Source: CAD feature listing. Evaluate the final solid. Frame: model axes, mm. Face numbers are marked on the shaded views. Round coordinates to 2 decimals unless told otherwise and drop trailing zeros. Loops run counter-clockwise (first coordinate to the right, second up) from the corner with the lowest first, then second, coordinate; pieces in that order, holes last. Notation, with made-up numbers: (66.5, -16.75) - (125.5, -16.75) arc R19 cw to (125.5, 8.25) - close; hole circle Ø10 at (29, -27). An arc over 180 degrees is marked (long way). Write item = value, one per line. Start each with the question number.
from build123d import *

# Parameters (mm, degrees)
F0_W      = 80
F0_H      = 120
F0_R      = 2.5
F0_R_2    = 1
F1_DEPTH  = 50
F3_DEPTH  = 120.001
F5_R      = 5
F6_DEPTH  = 10
F7_R      = 7.5
F8_DEPTH  = 120
F13_R     = 1
F15_DEPTH = 94.020238
F14_R     = 1
F16_DEPTH = 94.020238


with BuildPart() as f1:
    # F0 (on Front) → F1 (new body)
    with BuildSketch(Plane.XZ):
        Rectangle(F0_W, F0_H)
        with Locations((0, -50)):
            Circle(F0_R, mode=Mode.SUBTRACT)
        with Locations((0, 30)):
            Circle(F0_R, mode=Mode.SUBTRACT)
        with Locations((0, 45)):
            Circle(F0_R_2, mode=Mode.SUBTRACT)
    extrude(amount=F1_DEPTH)

    # F2 (on face) → F3 (cut, through all)
    with BuildSketch(Plane(origin=(0, 0, -60), x_dir=(1, 0, 0), z_dir=(0, 0, -1))):
        with BuildLine():
            Line((43.30127, 50), (-43.30127, 50))
            ThreePointArc((-43.30127, 50), (0, 25), (43.30127, 50))
        make_face()
    extrude(amount=-F3_DEPTH, mode=Mode.SUBTRACT)

    # F5 (on offset) → F6 (cut)
    with BuildSketch(Plane.XZ.offset(30)):
        with Locations((0, -50)):
            Circle(F5_R)
        with Locations((0, 30)):
            Circle(F5_R)
    extrude(amount=-F6_DEPTH, mode=Mode.SUBTRACT)

    # F7 (on face) → F8 (cut, through all)
    with BuildSketch(Plane(origin=(0, 0, -60), x_dir=(1, 0, 0), z_dir=(0, 0, -1))):
        with Locations((-17.5, 12)):
            Circle(F7_R)
        with Locations((17.5, 12)):
            Circle(F7_R)
    extrude(amount=-F8_DEPTH, mode=Mode.SUBTRACT)

    # F13 (on face) → F15 (cut, through all)
    with BuildSketch(Plane(origin=(17.524047, 30.35254, 0), x_dir=(-0.866025, 0.5, 0), z_dir=(0.5, 0.866025, 0))):
        with Locations((-37.5, 45)):
            Circle(F13_R)
    extrude(amount=-F15_DEPTH, mode=Mode.SUBTRACT)

    # F14 (on face) → F16 (cut, through all)
    with BuildSketch(Plane(origin=(-17.524047, 30.35254, 0), x_dir=(-0.866025, -0.5, 0), z_dir=(-0.5, 0.866025, 0))):
        with Locations((37.5, 45)):
            Circle(F14_R)
    extrude(amount=-F16_DEPTH, mode=Mode.SUBTRACT)


solid = f1.part
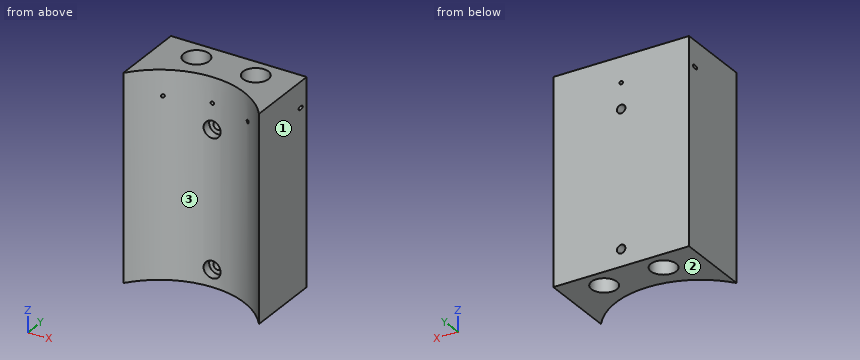
(1) Cut plane D-D (y = -17). State how many separate pieces and enclosed holes the cut face has, and give its area (3 significant figures).
(2) Material intervals for line 1 along Z through (x, y) = (0, -23); line 2 along X through (y, z) = (-11, 30); line 3 along X through (y, z) = (-21.15, -50), sorted ascending. Write a range as from..to.
(3) Cut plane B-B (z = -9.5). Output: boundary loops of the cut face in (x, y).
(4) Cut plane C-C (x = -15). Output: boundary loops of the cut face in (y, z), and give its area (3 significant figures).
(5) Mould query, pull axis X, two halves, no side actions, for the marked faces 1, 2 and 3. Classes: +X half, -X half, draft (parallel to the pull), parting line (faces both ways), or undercut.
(6) Pin query (flat end, axial travel): P1, Ø12, axis at x = -29, z = -19, coming from the -Y side; P2, Ø2, axis at x = -10, z = -32, coming from the -Y side (3 decimals); P3, Ø16, axis at x = 0, z = -50, coming from the -Y side. Return the tip coordinate at first contact, or that it passes through.
(7) Cut plane A-A (z = 30). Output: boundary loops of the cut face in (x, y).
Solution:
q1.separate_pieces = 3
q1.enclosed_holes = 5
q1.area = 6,870 mm^2
q2.line_1 = -60..-55, -45..25, 35..44, 46..60
q2.line_2 = -40..-24.93, -10.07..-2.5, 2.5..10.07, 24.93..40
q2.line_3 = -40..-5, 5..40
q3.outline = (-40, -45) arc R50 cw to (40, -45) - (40, 0) - (-40, 0) - close; hole circle Ø15 at (-17.5, -12); hole circle Ø15 at (17.5, -12)
q4.outline = (-27.3, -60) - (-19.07, -60) - (-19.07, 60) - (-27.3, 60) - close; (-4.93, -60) - (0, -60) - (0, 60) - (-4.93, 60) - close
q4.area = 1,580 mm^2
q5.face_1 = +X half
q5.face_2 = draft
q5.face_3 = undercut
q6.P1 = -39.29
q6.P2 = -26.225
q6.P3 = -25.64
q7.outline = (-40, -45) arc R50 cw to (-5, -25.25) - (-5, -20) - (-2.5, -20) - (-2.5, 0) - (-40, 0) - close; (2.5, -20) - (5, -20) - (5, -25.25) arc R50 cw to (40, -45) - (40, 0) - (2.5, 0) - close; hole circle Ø15 at (-17.5, -12); hole circle Ø15 at (17.5, -12)
